Can you work these out from the model? Positions are in its coordinate system, mm. Face numbers are marked on the shaded views. A direction names the side the tool comes from. Give positions to 0.01 mm unless a question says otherwise; leave off trailing zeros. Order: outer loops, then holes, each group sorted by start corner. A loop starts at its lowest first (then second) coordinate and runs counter-clockwise, first axis right, second up.
```python
from build123d import *

# Parameters (mm, degrees)
SKETCH1_W           = 70
SKETCH1_H           = 46
BOSS_EXTRUDE1_DEPTH = 5
SKETCH2_W           = 60
SKETCH2_H           = 30.5
CUT_EXTRUDE1_DEPTH  = 5
SKETCH3_W           = 70
SKETCH3_H           = 7.75
BOSS_EXTRUDE2_DEPTH = 8
CUT_EXTRUDE4_DEPTH  = 8.5
CUT_EXTRUDE5_DEPTH  = 8.5
CUT_EXTRUDE6_DEPTH  = 8.5


with BuildPart() as part:
    # Sketch1 → Boss-Extrude1 (new body)
    with BuildSketch(Plane(origin=(0, 0, 0), x_dir=(1, 0, 0), z_dir=(0, 1, 0))):
        Rectangle(SKETCH1_W, SKETCH1_H)
    extrude(amount=BOSS_EXTRUDE1_DEPTH)

    # Sketch2 → Cut-Extrude1 (cut)
    with BuildSketch(Plane(origin=(0, 0, 0), x_dir=(1, 0, 0), z_dir=(0, 1, 0))):
        Rectangle(SKETCH2_W, SKETCH2_H)
    extrude(amount=CUT_EXTRUDE1_DEPTH, mode=Mode.SUBTRACT)

    # Sketch3 → Boss-Extrude2 (add)
    with BuildSketch(Plane(origin=(0, 0, 0), x_dir=(1, 0, 0), z_dir=(0, 1, 0))):
        with Locations((0, -19.125)):
            Rectangle(SKETCH3_W, SKETCH3_H)
        with Locations((0, 19.125)):
            Rectangle(SKETCH3_W, SKETCH3_H)
    extrude(amount=-BOSS_EXTRUDE2_DEPTH)

    # Sketch6 → Cut-Extrude4 (cut)
    with BuildSketch(Plane.ZY.offset(35)):
        Polygon((19.125, -2.761751346), (21.625, -1.318375673), (21.625, 1.568375673), (19.125, 3.011751346), (16.625, 1.568375673), (16.625, -1.318375673), align=None)
        Polygon((-19.125, -2.761751346), (-16.625, -1.318375673), (-16.625, 1.568375673), (-19.125, 3.011751346), (-21.625, 1.568375673), (-21.625, -1.318375673), align=None)
    extrude(amount=-CUT_EXTRUDE4_DEPTH, mode=Mode.SUBTRACT)

    # Sketch7 → Cut-Extrude5 (cut)
    with BuildSketch(Plane(origin=(35, 0, 0), x_dir=(0, 0, -1), z_dir=(1, 0, 0))):
        Polygon((-19.125, -2.761751346), (-16.625, -1.318375673), (-16.625, 1.568375673), (-19.125, 3.011751346), (-21.625, 1.568375673), (-21.625, -1.318375673), align=None)
        Polygon((19.125, -2.761751346), (21.625, -1.318375673), (21.625, 1.568375673), (19.125, 3.011751346), (16.625, 1.568375673), (16.625, -1.318375673), align=None)
    extrude(amount=-CUT_EXTRUDE5_DEPTH, mode=Mode.SUBTRACT)

    # Sketch10 → Cut-Extrude6 (cut)
    with BuildSketch(Plane(origin=(0, 5, 0), x_dir=(1, 0, 0), z_dir=(0, 1, 0))):
        Polygon((2.886751346, 18.835), (1.443375673, 21.335), (-1.443375673, 21.335), (-2.886751346, 18.835), (-1.443375673, 16.335), (1.443375673, 16.335), align=None)
        Polygon((2.886751346, -18.835), (1.443375673, -16.335), (-1.443375673, -16.335), (-2.886751346, -18.835), (-1.443375673, -21.335), (1.443375673, -21.335), align=None)
    extrude(amount=-CUT_EXTRUDE6_DEPTH, mode=Mode.SUBTRACT)


solid = part.part
```
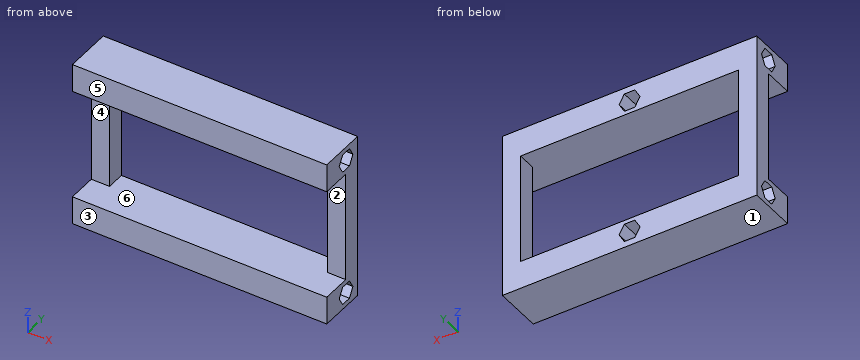
1) We'd pull the mould along Z, two halves only. Please class the marked faces 1, 2 and 3: +Z half, -Z half, draft (parallel to the pull), parting line (faces both ways), or undercut.
2) I'm going to push flat-ended pins straight in: pin 1 Ø4 at (x, z) = (-32, 0) entering from -Y; pin 2 Ø1 at (x, z) = (-27, 13) entering from -Y; pin 3 Ø1.5 at (x, z) = (0, -20) entering from +Y. Where does each tip first touch, or does it pass through?
3) Suppose I cut it at C-C (y = 2.25). Give the number of separate pieces and of enclosed holes in the cut face, and give its area (3 significant figures).
4) If I drill on line 1 (X direction, y = 1, z = 9); line 2 (Z direction, x = -23.5, y = 1.25); line 3 (Z direction, x = 29.5, y = -2.25), over which ranges is the centre line in solid material (lowest first)?
5) Which directions (+Z, -Z, +X, -X, +Y, -Y) give clear straight access to the entire face, cutting with the end or side of a thin tool? Please do the marked faces 4, 5 and 6.
6) Suppose I cut it at A-A (z = 9). Please give me the cut outline in (x, y).
7) Suppose I cut it at B-B (x = 22). Please give me the cut outline in (y, z), and give its area (4 significant figures).
Results:
1. face 1: -Z half
1. face 2: undercut
1. face 3: draft
2. pin 1: stops at y = 0
2. pin 2: passes through
2. pin 3: stops at y = -3.5
3. separate pieces: 1
3. enclosed holes: 3
3. area: 1,260 mm2
4. line 1: x = -35 to -30, 30 to 35
4. line 2: z = -23 to -15.25, 15.25 to 23
4. line 3: z = -23 to -20.01, -18.24 to -15.25, 15.25 to 18.24, 20.01 to 23
5. face 4: +X, -X, -Y
5. face 5: +Z, -Z, +X, -X, -Y
5. face 6: -Y
6. outline: (-35, 0) - (-30, 0) - (-30, 5) - (-35, 5) - close; (30, 0) - (35, 0) - (35, 5) - (30, 5) - close
7. outline: (-8, -23) - (5, -23) - (5, -15.25) - (-8, -15.25) - close; (-8, 15.25) - (5, 15.25) - (5, 23) - (-8, 23) - close
7. area: 201.5 mm2
